The listing builds one solid part. Answer for the finished solid, in the listing's coordinates (mm). A direction names the side the tool comes from. Give positions to 0.01 mm unless a question says otherwise; leave off trailing zeros. Write each loop counter-clockwise with the first axis right and the second up, starting at its lowest first coordinate (ties: lowest second). Pieces come first, ordered by that corner, then holes. Notation, with made-up numbers: (55.5, -7) - (66.5, -7) arc R25 ccw to (66.5, 7) - close; hole circle Ø11 at (84.5, -2). An arc over 180 degrees is marked (long way). Return JSON: item names as keys, results as strings.
from build123d import *

# Parameters (mm, degrees)
SKETCH1_W           = 62
SKETCH1_H           = 78
BOSS_EXTRUDE1_DEPTH = 2
SKETCH2_W           = 62
SKETCH2_H           = 78
SKETCH2_W_2         = 58
SKETCH2_H_2         = 64
BOSS_EXTRUDE2_DEPTH = 20
CUT_EXTRUDE1_REACH  = 86.481
SKETCH3_R           = 3.313142946
SKETCH4_W           = 62
SKETCH4_H           = 27
BOSS_EXTRUDE3_DEPTH = 2
SKETCH5_W           = 2
SKETCH5_H           = 27
BOSS_EXTRUDE4_DEPTH = 20
SKETCH6_W           = 58
SKETCH6_H           = 27
BOSS_EXTRUDE5_DEPTH = 2
SKETCH9_W           = 57.873853322
SKETCH9_H           = 10
CUT_EXTRUDE4_DEPTH  = 14.5
SKETCH12_W          = 58
SKETCH12_H          = 27
BOSS_EXTRUDE6_DEPTH = 3
SKETCH13_W          = 58
SKETCH13_H          = 92.14389058
CUT_EXTRUDE6_DEPTH  = 3
CUT_EXTRUDE7_REACH  = 77.353
SKETCH14_W          = 9.5
SKETCH14_H          = 6


with BuildPart() as part:
    # Sketch1 → Boss-Extrude1 (new body)
    with BuildSketch(Plane.XY):
        Rectangle(SKETCH1_W, SKETCH1_H)
    extrude(amount=-BOSS_EXTRUDE1_DEPTH)

    # Sketch2 → Boss-Extrude2 (add)
    with BuildSketch(Plane.XY):
        Rectangle(SKETCH2_W, SKETCH2_H)
        with Locations((0, 5)):
            Rectangle(SKETCH2_W_2, SKETCH2_H_2, mode=Mode.SUBTRACT)
    extrude(amount=BOSS_EXTRUDE2_DEPTH)

    # Sketch3 → Cut-Extrude1 (cut, up to next)
    with BuildSketch(Plane.XZ.offset(-37), mode=Mode.PRIVATE) as cut_extrude1_sk1:
        with Locations((-20.488158498, 8.767623766)):
            Circle(SKETCH3_R)
    cut_extrude1_tool1 = extrude(cut_extrude1_sk1.sketch, amount=-CUT_EXTRUDE1_REACH, mode=Mode.PRIVATE) & part.part
    add(cut_extrude1_tool1.solids().sort_by_distance((-20.488158, 37, 8.767624))[0], mode=Mode.SUBTRACT)

    # Sketch4 → Boss-Extrude3 (add)
    with BuildSketch(Plane.XY):
        with Locations((0, 52.5)):
            Rectangle(SKETCH4_W, SKETCH4_H)
    extrude(amount=-BOSS_EXTRUDE3_DEPTH)

    # Sketch5 → Boss-Extrude4 (add)
    with BuildSketch(Plane.XY):
        with Locations((-30, 52.5)):
            Rectangle(SKETCH5_W, SKETCH5_H)
        with Locations((30, 52.5)):
            Rectangle(SKETCH5_W, SKETCH5_H)
    extrude(amount=BOSS_EXTRUDE4_DEPTH)

    # Sketch6 → Boss-Extrude5 (add)
    with BuildSketch(Plane.XY.offset(20)):
        with Locations((0, 52.5)):
            Rectangle(SKETCH6_W, SKETCH6_H)
    extrude(amount=-BOSS_EXTRUDE5_DEPTH)

    # Sketch9 → Cut-Extrude4 (cut)
    with BuildSketch(Plane.XY):
        with Locations((-0.063073339, -34)):
            Rectangle(SKETCH9_W, SKETCH9_H)
    extrude(amount=CUT_EXTRUDE4_DEPTH, mode=Mode.SUBTRACT)

    # Sketch12 → Boss-Extrude6 (add)
    with BuildSketch(Plane(origin=(0, 0, 18), x_dir=(-1, 0, 0), z_dir=(0, 0, -1))):
        with Locations((0, 52.5)):
            Rectangle(SKETCH12_W, SKETCH12_H)
    extrude(amount=BOSS_EXTRUDE6_DEPTH)

    # Sketch13 → Cut-Extrude6 (cut)
    with BuildSketch(Plane.XY.offset(20)):
        with Locations((0, 7.07194529)):
            Rectangle(SKETCH13_W, SKETCH13_H)
    extrude(amount=-CUT_EXTRUDE6_DEPTH, mode=Mode.SUBTRACT)

    # Cut-Extrude7: up to this face of the body (flat: up to its plane)
    cut_extrude7_end = Plane(part.part.faces().sort_by_distance((-0.063073339, -34, 0))[0])
    # Sketch14 → Cut-Extrude7 (cut, up to the picked face)
    with BuildSketch(Plane.XY.offset(17), mode=Mode.PRIVATE) as cut_extrude7_sk1:
        with Locations((0, 45.439187808)):
            Rectangle(SKETCH14_W, SKETCH14_H)
    cut_extrude7_tool1 = split(extrude(cut_extrude7_sk1.sketch, amount=-CUT_EXTRUDE7_REACH, mode=Mode.PRIVATE), bisect_by=cut_extrude7_end, keep=Keep.BOTH, mode=Mode.PRIVATE)
    # Sketch14 → Cut-Extrude7 (cut, up to the picked face)
    with BuildSketch(Plane.XY.offset(17), mode=Mode.PRIVATE) as cut_extrude7_sk2:
        with Locations((0, -33.160812192)):
            Rectangle(SKETCH14_W, SKETCH14_H)
    cut_extrude7_tool2 = split(extrude(cut_extrude7_sk2.sketch, amount=-CUT_EXTRUDE7_REACH, mode=Mode.PRIVATE), bisect_by=cut_extrude7_end, keep=Keep.BOTH, mode=Mode.PRIVATE)
    add(cut_extrude7_tool1.solids().sort_by(Axis((0, 45.439188, 17), (0, 0, -1)))[0], mode=Mode.SUBTRACT)
    add(cut_extrude7_tool2.solids().sort_by(Axis((0, -33.160812, 17), (0, 0, -1)))[0], mode=Mode.SUBTRACT)


solid = part.part
Item 1: A cutting plane is placed at A-A on z = 2.5. Determine the outline of the cut face in (x, y), then the cut area to 3 significant figures.
Answer below:
{"outline": "(-31, -39) - (-29, -39) - (-29, -29) - (28.87, -29) - (28.87, -39) - (31, -39) - (31, 66) - (29, 66) - (29, 39) - (-29, 39) - (-29, 66) - (-31, 66) - close; hole (-29, -27) - (29, -27) - (29, 37) - (-29, 37) - close", "area": "653 mm²"}
Item 2: Consider L1, parallel to Y at x = -2.5, z = 16; L2, parallel to Y at x = -15.5, z = 6.75; L3, parallel to X at y = 17, z = 1.5. Determine where each line is inside the solid, lowest interval first.
Answer below:
{"L1": "y = -39 to -36.16, -30.16 to -27, 37 to 42.44, 48.44 to 66", "L2": "y = -29 to -27, 37 to 39", "L3": "x = -31 to -29, 29 to 31"}
Item 3: A cutting plane is placed at B-B on y = 3.5. Determine the outline of the cut face in (x, z).
Answer below:
{"outline": "(-31, -2) - (31, -2) - (31, 20) - (29, 20) - (29, 0) - (-29, 0) - (-29, 20) - (-31, 20) - close"}
Item 4: A cutting plane is placed at C-C on x = 3. Determine the outline of the cut face in (y, z), then the cut area to 3 significant figures.
Answer below:
{"outline": "(-39, -2) - (66, -2) - (66, 0) - (39, 0) - (39, 15) - (42.44, 15) - (42.44, 17) - (37, 17) - (37, 0) - (-27, 0) - (-27, 17) - (-30.16, 17) - (-30.16, 14.5) - (-29, 14.5) - (-29, 0) - (-39, 0) - close; (-39, 14.5) - (-36.16, 14.5) - (-36.16, 17) - (-39, 17) - close; (48.44, 15) - (66, 15) - (66, 20) - (53.14, 20) - (53.14, 17) - (48.44, 17) - close", "area": "369 mm²"}
Item 5: Flat-ended cylindrical pins translate along their axes: P1, Ø8, axis at x = 8.5, y = 48.5, coming from the +Z side; P2, Ø1, axis at x = -10.5, z = 7, coming from the +Y side; P3, Ø0.9, axis at x = -1, z = 18, coming from the -Y side. Find the tip coordinate at first contact, or state that the pin passes through.
Answer below:
{"P1": "stops at z = 17", "P2": "stops at y = 39", "P3": "stops at y = 53.14"}
Item 6: For faces 1 (the face through (0, 53, 15)), 2 (the face through (0, -37, 17)), 3 (the face through (0, -37, 14.5)), 4 (the face through (-4.75, -33, 16)), determine the directions among +Z, -Z, +X, -X, +Y, -Y from which every point of the face is accessible in a straight line to the end or side of a thin tool.
Answer below:
{"face 1": "+Y", "face 2": "+Z, -Y", "face 3": "-Y", "face 4": "+Z"}
Item 7: The mould has two halves that part along Y. Classify faces 5 (the face through (0, 66, 16)), 6 (the face through (0, 49, 17)), 7 (the face through (0, -30.161, 16)): +Y half, -Y half, draft (parallel to the pull), parting line (faces both ways), or undercut.
Answer below:
{"face 5": "+Y half", "face 6": "draft", "face 7": "undercut"}
Item 8: A cutting plane is placed at D-D on y = 59.5. Determine the outline of the cut face in (x, z).
Answer below:
{"outline": "(-31, -2) - (31, -2) - (31, 20) - (-31, 20) - close; hole (-29, 0) - (29, 0) - (29, 15) - (-29, 15) - close"}
